Check sheet for the modelled part. Datum: model origin and axes. Units: mm. A direction names the side the tool comes from. Round coordinates to 2 decimals unless told otherwise and drop trailing zeros. Write each loop counter-clockwise with the first axis right and the second up, starting at its lowest first coordinate (ties: lowest second). Pieces come first, ordered by that corner, then holes. Notation, with made-up numbers: (-22.5, 35) -> (-13.5, 35) arc R17 cw to (-13.5, 48) -> close; hole circle Ø5 at (-24.75, 40.25). An arc over 180 degrees is marked (long way). One line per item, written item: value.
from build123d import *

# Parameters (mm, degrees)
EXTRUDE_THIN4_DEPTH     = 10
SKETCH2_R               = 1.25
CUT_EXTRUDE1_DEPTH      = 20.798989873
MIRROR2_COPY_1_SKETCH_R = 1.25
MIRROR2_COPY_1_DEPTH    = 20.798989873


with BuildPart() as part:
    # Sketch1 → Extrude-Thin4 (new body)
    with BuildSketch(Plane.XY):
        with BuildLine():
            Line((0, 0), (-5, 0))
            Line((-5, 0), (-5, -3))
            ThreePointArc((-5, -3), (-8, -6), (-11, -3))
            Line((-11, -3), (-11, 0))
            Line((-11, 0), (-16, 0))
            Line((-16, 0), (-16, 0.5))
            Line((-16, 0.5), (-10.5, 0.5))
            Line((-10.5, 0.5), (-10.5, -3))
            ThreePointArc((-10.5, -3), (-8, -5.5), (-5.5, -3))
            Line((-5.5, -3), (-5.5, 0.5))
            Line((-5.5, 0.5), (0, 0.5))
            Line((0, 0.5), (0, 0))
        make_face()
    extrude(amount=EXTRUDE_THIN4_DEPTH)

    # Sketch2 → Cut-Extrude1 (cut, through all)
    with BuildSketch(Plane(origin=(0, 0, 0), x_dir=(1, 0, 0), z_dir=(0, 1, 0))):
        with Locations(Location((-13.110421324, -2.595753644, 0), (0, 0, 270))):
            Circle(SKETCH2_R)
    cut_extrude1 = extrude(amount=CUT_EXTRUDE1_DEPTH, mode=Mode.SUBTRACT)

    # Mirror1: Cut-Extrude1 across plane
    add(cut_extrude1.mirror(Plane.XY.offset(5)), mode=Mode.SUBTRACT)

    # Mirror2: Cut-Extrude1 across plane
    add(cut_extrude1.mirror(Plane(origin=(-8, 0, 0), x_dir=(0, 0, 1), z_dir=(1, 0, 0))), mode=Mode.SUBTRACT)

    # Mirror2 copy 1 sketch → Mirror2 copy 1 (cut, through all)
    with BuildSketch(Plane(origin=(-16, 0, 10), x_dir=(-1, 0, 0), z_dir=(0, 1, 0))):
        with Locations(Location((-13.110421324, -2.595753644, 0), (0, 0, 270))):
            Circle(MIRROR2_COPY_1_SKETCH_R)
    extrude(amount=MIRROR2_COPY_1_DEPTH, mode=Mode.SUBTRACT)


solid = part.part
Item 1: Depth check by flat-ended pin: P1, Ø0.9, axis at y = -2, z = 5.5, coming from the -X side; P2, Ø3, axis at x = -2.89, z = 2.6, coming from the -Y side; P3, Ø1.5, axis at y = -1.5, z = 6.5, coming from the +X side. Enter the tip coordinate at first touch or a pass-through.
Answer:
P1: stops at x = -11
P2: stops at y = 0
P3: stops at x = -5
Item 2: Tool access check on faces 5 (the flat face through (-13, 0, 5)), 6 (the flat face through (-10.5, -1, 5)), 7 (the flat face through (-5, -1, 5)), 8 (the cylindrical face through (-11.87, 0.25, 7.57)). Record the directions out of +Z, -Z, +X, -X, +Y, -Y that give a thin tool (end or side, any length) a straight path to the whole face; none if there is none.
Answer:
face 5: +Z, -Z, -X, -Y
face 6: +Z, -Z, +Y
face 7: +Z, -Z, +X, -Y
face 8: +Y, -Y
Item 3: Sectioned sample at D-D on x = -8. Enter the section's corners in (y, z), and give its area (3 significant figures).
Answer:
outline: (-6, 0) -> (-5.5, 0) -> (-5.5, 10) -> (-6, 10) -> close
area: 5.00 mm^2
Item 4: Sectioned sample at B-B on z = 3.25. Enter the section's corners in (x, y), and give its area (3 significant figures).
Answer:
outline: (-16, 0) -> (-14.18, 0) -> (-14.18, 0.5) -> (-16, 0.5) -> close; (-12.05, 0) -> (-11, 0) -> (-11, -3) arc R3 ccw to (-5, -3) -> (-5, 0) -> (-3.95, 0) -> (-3.95, 0.5) -> (-5.5, 0.5) -> (-5.5, -3) arc R2.5 cw to (-10.5, -3) -> (-10.5, 0.5) -> (-12.05, 0.5) -> close; (-1.82, 0) -> (0, 0) -> (0, 0.5) -> (-1.82, 0.5) -> close
area: 10.7 mm^2
Item 5: Thickness scan on line 1 (X direction, y = -1, z = 6.5); line 2 (Y direction, x = -11.5, z = 4.75); line 3 (X direction, y = -4, z = 5). Record the ranges inside material, lowest first.
Answer:
line 1: x = -11 to -10.5, -5.5 to -5
line 2: y = 0 to 0.5
line 3: x = -10.83 to -10.29, -5.71 to -5.17
Item 6: Mould release check, pull along X, two halves, no side actions. Record for faces 1 (the flat face through (-11, -2, 5)), 2 (the cylindrical face through (-2.945, 0.246, 8.653)), 3 (the flat face through (-2, 0, 5)), 4 (the flat face through (-5.5, -1, 5)): pulls with the +X half, pulls with the -X half, needs draft (parallel to the pull), parting line crosses it, or undercut.
Answer:
face 1: pulls with the -X half
face 2: undercut
face 3: needs draft
face 4: undercut
Item 7: Sectioned sample at C-C on z = 5.75. Enter the section's corners in (x, y), and give its area (3 significant figures).
Answer:
outline: (-16, 0) -> (-11, 0) -> (-11, -3) arc R3 ccw to (-5, -3) -> (-5, 0) -> (0, 0) -> (0, 0.5) -> (-5.5, 0.5) -> (-5.5, -3) arc R2.5 cw to (-10.5, -3) -> (-10.5, 0.5) -> (-16, 0.5) -> close
area: 12.8 mm^2
Item 8: Sectioned sample at A-A on y = -0.75. Enter the section's corners in (x, z).
Answer:
outline: (-11, 0) -> (-10.5, 0) -> (-10.5, 10) -> (-11, 10) -> close; (-5.5, 0) -> (-5, 0) -> (-5, 10) -> (-5.5, 10) -> close
